Check sheet for the modelled part. Datum: model origin and axes. Units: mm. Face numbers are marked on the shaded views. Round coordinates to 2 decimals unless told otherwise and drop trailing zeros. Write each loop counter-clockwise with the first axis right and the second up, starting at its lowest first coordinate (ties: lowest second). Pieces come first, ordered by that corner, then holes. Notation, with made-up numbers: M 0.25,29.25 L 20.25,29.25 A17 cw 20.25,43.25 Z; hole C 61.25,-8 d8. An arc over 180 degrees is marked long. Answer in a Markdown table with one row per item.
```python
from build123d import *

# Parameters (mm, degrees)
SKETCH_W        = 70
SKETCH_H        = 50
PAD_DEPTH       = 5
SKETCH001_R     = 2.625
POCKET_DEPTH    = 5
SKETCH002_W     = 47
SKETCH002_H     = 50
PAD001_DEPTH    = 50
SKETCH003_W     = 36.5
SKETCH003_H     = 50
POCKET001_DEPTH = 50
POCKET002_DEPTH = 40
POCKET003_DEPTH = 50
SKETCH005_W     = 5.25
SKETCH005_H     = 55
PAD002_DEPTH    = 53
SKETCH006_R     = 1.75
POCKET004_DEPTH = 7
SKETCH007_R     = 11.5
POCKET005_DEPTH = 3
SKETCH008_R     = 2.75
POCKET006_DEPTH = 4
SKETCH009_R     = 2.625
POCKET007_DEPTH = 5
SKETCH010_W     = 40
SKETCH010_H     = 5
PAD003_DEPTH    = 40
SKETCH011_R     = 2.625
POCKET008_DEPTH = 5
SKETCH012_W     = 30
SKETCH012_H     = 5
PAD004_DEPTH    = 10


with BuildPart() as part:
    # Sketch → Pad (new body)
    with BuildSketch(Plane.XY):
        Rectangle(SKETCH_W, SKETCH_H)
    extrude(amount=PAD_DEPTH)

    # Sketch001 (on Face6 of Pad) → Pocket (cut)
    with BuildSketch(Plane.XY.offset(5)):
        with Locations((-30, 20)):
            Circle(SKETCH001_R)
        with Locations((30, 20)):
            Circle(SKETCH001_R)
        with Locations((30, -20)):
            Circle(SKETCH001_R)
        with Locations((-30, -20)):
            Circle(SKETCH001_R)
    extrude(amount=-POCKET_DEPTH, mode=Mode.SUBTRACT)

    # Sketch002 (on Face5 of Pocket) → Pad001 (join)
    with BuildSketch(Plane.XY.offset(5)):
        Rectangle(SKETCH002_W, SKETCH002_H)
    extrude(amount=PAD001_DEPTH)

    # Sketch003 (on Face16 of Pad001) → Pocket001 (cut)
    with BuildSketch(Plane.XY.offset(55)):
        Rectangle(SKETCH003_W, SKETCH003_H)
    extrude(amount=-POCKET001_DEPTH, mode=Mode.SUBTRACT)

    # Sketch004 (on Face18 of Pocket001) → Pocket002 (cut)
    with BuildSketch(Plane.YZ.offset(23.5)):
        with BuildLine():
            Line((-8.332745, 55), (-1.252745, 47.92))
            ThreePointArc((-7.08, 42.08), (-1.246373, 42.086373), (-1.252745, 47.92))
            Line((-20, 55), (-7.08, 42.08))
            Line((-20, 55), (-8.332745, 55))
        make_face()
    extrude(amount=-POCKET002_DEPTH, mode=Mode.SUBTRACT)

    # Sketch004 (on Face18 of Pocket001) → Pocket003 (cut)
    with BuildSketch(Plane.YZ.offset(23.5)):
        with BuildLine():
            Line((-8.332745, 55), (-1.252745, 47.92))
            ThreePointArc((-7.08, 42.08), (-1.246373, 42.086373), (-1.252745, 47.92))
            Line((-20, 55), (-7.08, 42.08))
            Line((-20, 55), (-8.332745, 55))
        make_face()
    extrude(amount=-POCKET003_DEPTH, mode=Mode.SUBTRACT)

    # Sketch005 (on Face8 of Pocket003) → Pad002 (join)
    with BuildSketch(Plane.XZ.offset(25)):
        with Locations((20.875, 27.5)):
            Rectangle(SKETCH005_W, SKETCH005_H)
    extrude(amount=PAD002_DEPTH)

    # Sketch006 (on Face28 of Pad002) → Pocket004 (cut)
    with BuildSketch(Plane.YZ.offset(23.5)):
        with Locations((-73, 50)):
            Circle(SKETCH006_R)
        with Locations((-42, 50)):
            Circle(SKETCH006_R)
        with Locations((-42, 19)):
            Circle(SKETCH006_R)
        with Locations((-73, 19)):
            Circle(SKETCH006_R)
    extrude(amount=-POCKET004_DEPTH, mode=Mode.SUBTRACT)

    # Sketch007 (on Face32 of Pocket004) → Pocket005 (cut)
    with BuildSketch(Plane.YZ.offset(23.5)):
        with Locations((-57.5, 34.5)):
            Circle(SKETCH007_R)
    extrude(amount=-POCKET005_DEPTH, mode=Mode.SUBTRACT)

    # Sketch008 (on Face8 of Pocket005) → Pocket006 (cut)
    with BuildSketch(Plane(origin=(18.25, 0, 0), x_dir=(0, -1, 0), z_dir=(-1, 0, 0))):
        with Locations((42, 50)):
            Circle(SKETCH008_R)
        with Locations((73, 50)):
            Circle(SKETCH008_R)
        with Locations((73, 19)):
            Circle(SKETCH008_R)
        with Locations((42, 19)):
            Circle(SKETCH008_R)
    extrude(amount=-POCKET006_DEPTH, mode=Mode.SUBTRACT)

    # Sketch009 (on Face49 of Pocket006) → Pocket007 (cut)
    with BuildSketch(Plane.YZ.offset(20.5)):
        with Locations((-57.5, 34.5)):
            Circle(SKETCH009_R)
    extrude(amount=-POCKET007_DEPTH, mode=Mode.SUBTRACT)

    # Sketch010 (on Face3 of Pocket007) → Pad003 (join)
    with BuildSketch(Plane(origin=(0, 25, 0), x_dir=(-1, 0, 0), z_dir=(0, 1, 0))):
        with Locations((15, 2.5)):
            Rectangle(SKETCH010_W, SKETCH010_H)
    extrude(amount=PAD003_DEPTH)

    # Sketch011 (on Face10 of Pad003) → Pocket008 (cut)
    with BuildSketch(Plane.XY.offset(5)):
        with Locations((-30, 60)):
            Circle(SKETCH011_R)
        with Locations((-10, 60)):
            Circle(SKETCH011_R)
    extrude(amount=-POCKET008_DEPTH, mode=Mode.SUBTRACT)

    # Sketch012 (on Face14 of Pocket008) → Pad004 (join)
    with BuildSketch(Plane(origin=(0, 25, 0), x_dir=(-1, 0, 0), z_dir=(0, 1, 0))):
        with Locations((-20, 2.5)):
            Rectangle(SKETCH012_W, SKETCH012_H)
    extrude(amount=PAD004_DEPTH)


solid = part.part
```
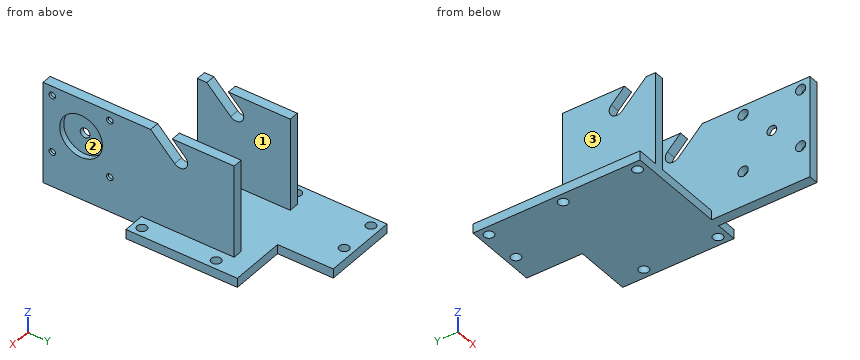
1. Scan lines: L1, parallel to X at y = 9.5, z = 47; L2, parallel to Z at x = 20.6, y = -73; L3, parallel to Z at x = 18.95, y = -57.5 (3 decimals). Record each from-to range of solid material in increasing order.
Found:
| item | result |
|---|---|
| L1 | x = -23.5 to -18.25, 18.25 to 23.5 |
| L2 | z = 0 to 16.25, 21.75 to 47.25, 52.75 to 55 |
| L3 | z = 0 to 31.875, 37.125 to 55 |
2. Section check B-B, the plane x = -30. Record the cut outline in (y, z) (3 decimals), and give its area (3 significant figures).
Found:
| item | result |
|---|---|
| outline | M -25,0 L -22.625,0 L -22.625,5 L -25,5 Z; M -17.375,0 L 17.375,0 L 17.375,5 L -17.375,5 Z; M 22.625,0 L 57.375,0 L 57.375,5 L 22.625,5 Z; M 62.625,0 L 65,0 L 65,5 L 62.625,5 Z |
| area | 371 mm2 |
3. Section check D-D, the plane x = -10. Record the cut outline in (y, z) (3 decimals).
Found:
| item | result |
|---|---|
| outline | M -25,0 L 57.375,0 L 57.375,5 L -25,5 Z; M 62.625,0 L 65,0 L 65,5 L 62.625,5 Z |
4. Go/stop test with flat-tipped pins: pin 1 (2 mm diameter, centred on y = 9.5, z = 30, fed in from +X); pin 2 (1.6 mm diameter, centred on x = -20.5, z = 24, fed in from +Y); pin 3 (5 mm diameter, centred on y = -3.5, z = 39.5, fed in from -X). Record where each tip stops, or that it passes through.
Found:
| item | result |
|---|---|
| pin 1 | stops at x = 23.5 |
| pin 2 | stops at y = 25 |
| pin 3 | stops at x = -23.5 |
5. Draft check along X on the marked faces 1, 2 and 3. Enter one of: +X half, -X half, draft (parallel to the pull), parting line (faces both ways), or undercut.
Found:
| item | result |
|---|---|
| face 1 | undercut |
| face 2 | +X half |
| face 3 | -X half |
6. Section check A-A, the plane y = -57.5. Record the cut outline in (x, z) (3 decimals), and give its area (3 significant figures).
Found:
| item | result |
|---|---|
| outline | M 18.25,0 L 23.5,0 L 23.5,23 L 20.5,23 L 20.5,31.875 L 18.25,31.875 Z; M 18.25,37.125 L 20.5,37.125 L 20.5,46 L 23.5,46 L 23.5,55 L 18.25,55 Z |
| area | 208 mm2 |
7. Section check C-C, the plane z = 25. Record the cut outline in (x, y).
Found:
| item | result |
|---|---|
| outline | M -23.5,-25 L -18.25,-25 L -18.25,25 L -23.5,25 Z; M 18.25,-78 L 23.5,-78 L 23.5,-63.98 L 20.5,-63.98 L 20.5,-51.02 L 23.5,-51.02 L 23.5,25 L 18.25,25 Z |
